Can you work these out from the model? Positions are in its coordinate system, mm. A direction names the side the tool comes from. Give positions to 0.01 mm unless a question says otherwise; leave off trailing zeros. Write each loop counter-clockwise with the first axis right and the second up, starting at its lowest first coordinate (ties: lowest second). Pieces come first, ordered by that corner, then holes.
```python
from build123d import *

# Parameters (mm, degrees)
BOSS_EXTRUDE1_DEPTH      = 10
BOSS_EXTRUDE1_DEPTH_BACK = 10
CIRPATTERN1_COUNT        = 3


with BuildPart() as part:
    # Sketch2 → Boss-Extrude1 (new body, two sides)
    with BuildSketch(Plane.XY) as boss_extrude1_sk:
        Polygon((-10, 5.773502692), (10, 5.773502692), (0, -11.547005384), align=None)
    extrude(amount=BOSS_EXTRUDE1_DEPTH)
    extrude(boss_extrude1_sk.sketch, amount=-BOSS_EXTRUDE1_DEPTH_BACK)

    # Sketch2_7 → Revolve3 (revolve)
    with BuildSketch(Plane.XY):
        with BuildLine():
            Line((0, 9.982895082), (0, 5.773502692))
            Line((0, 5.773502692), (10, 5.773502692))
            ThreePointArc((10, 5.773502692), (5.424918992, 8.887653347), (0, 9.982895082))
        make_face()
    revolve3 = revolve(axis=Axis((0, 9.982895082, 0), (0, -1, 0)))

    # CirPattern1: Revolve3 ×3 about axis
    cirpattern1_axis = Axis((0, 0, 0), (0, 0, 1))
    for i in range(1, CIRPATTERN1_COUNT):
        add(revolve3.rotate(cirpattern1_axis, i * 360 / CIRPATTERN1_COUNT))


solid = part.part
```
1) Suppose I cut it at C-C on y = -0.5. Write out the boundary of the cut face in (x, z), plus the area to 3 significant figures.
Values follow:
outline: (-6.38, -10) - (6.38, -10) - (6.38, -9.61) arc R13.76 ccw to (6.38, 9.61) - (6.38, 10) - (-6.38, 10) - (-6.38, 9.61) arc R13.76 ccw to (-6.38, -9.61) - close
area: 359 mm2
2) Suppose I cut it at D-D on z = 2.75. Write out the boundary of the cut face in (x, y), plus the area to 3 significant figures.
Values follow:
outline: (-10, 5.77) - (-9.81, 5.44) arc R13.71 ccw to (-0.19, -11.21) - (0, -11.55) - (0.19, -11.21) arc R13.71 ccw to (9.81, 5.44) - (10, 5.77) - (9.61, 5.77) arc R13.71 ccw to (-9.61, 5.77) - close
area: 330 mm2
3) For faces 1 (the face through (-8, 5.774, -8)), 2 (the face through (8, 5.774, 8)), 3 (the face through (8, 5.774, -8)), 4 (the face through (1.215, -9.442, 7.986)), which set-ups out of +Z, -Z, +X, -X, +Y, -Y let a thin tool reach every point of the face, with its end or its side?
Values follow:
face 1: -Z, -X, +Y
face 2: +Z, +X, +Y
face 3: -Z, +X, +Y
face 4: +Z, +X, -Y
4) Suppose I cut it at B-B on x = 7.5. Write out the boundary of the cut face in (y, z), plus the area to 3 significant figures.
Values follow:
outline: (1.44, -10) - (5.77, -10) - (5.77, -6.61) arc R11.8 ccw to (5.77, 6.61) - (5.77, 10) - (1.44, 10) - (1.44, 8.66) arc R8.68 ccw to (1.44, -8.66) - close
area: 213 mm2
5) For pin 1 Ø1.5 at (x, y) = (-5, 7) entering from +Z; pin 2 Ø3 at (x, z) = (5, 6.5) entering from +Y; pin 3 Ø5 at (x, z) = (3, 5) entering from +Y, each with a flat end and sliding along its axis, tell me the tip position at first contact or that it passes through.
Values follow:
pin 1: stops at z = 8.19
pin 2: stops at y = 8.27
pin 3: stops at y = 9.58
6) Suppose I cut it at A-A on z = -3.25. Write out the boundary of the cut face in (x, y), plus the area to 3 significant figures.
Values follow:
outline: (-10, 5.77) - (-9.73, 5.3) arc R13.6 ccw to (-0.27, -11.08) - (0, -11.55) - (0.27, -11.08) arc R13.6 ccw to (9.73, 5.3) - (10, 5.77) - (9.46, 5.77) arc R13.6 ccw to (-9.46, 5.77) - close
area: 323 mm2
7) Please list where these lines run through material, in increasing order: L1, parallel to X at y = 2.25, z = -1.25; L2, parallel to Y at x = -1.25, z = -5; L3, parallel to X at y = -7.25, z = -1.
Values follow:
L1: x = -10.46 to 10.46
L2: y = -10.18 to 9
L3: x = -6.97 to 6.97
